CAD build for the part. Positions are in the model's coordinates, mm. Round coordinates to 2 decimals unless told otherwise and drop trailing zeros. Write each loop counter-clockwise with the first axis right and the second up, starting at its lowest first coordinate (ties: lowest second). Pieces come first, ordered by that corner, then holes. Notation, with made-up numbers: (76.25, 55) - (108.25, 55) arc R7 ccw to (108.25, 67) - close; hole circle Ø1 at (71, 10). An arc over 180 degrees is marked (long way). Answer in a Markdown table with one row per item.
Autodesk Inventor part; units mm, degrees
ref_plane "YZ Plane" through (0, 0, 0) normal (1, 0, 0) x (0, 1, 0)
ref_plane "XZ Plane" through (0, 0, 0) normal (0, 1, 0) x (-1, 0, 0)
ref_plane "XY Plane" through (0, 0, 0) normal (0, 0, 1) x (1, 0, 0)
sketch "Sketch1" plane through (0, 0, 0) normal (0, 1, 0) x (-1, 0, 0)
  circle A0 centre (64.977, -75.4393) radius 17
  line L0 (64.977, -75.4393) -> (99.977, -75.4393)
  line L1 (64.977, -75.4393) -> (47.477, -45.1285)
  line L2 (64.977, -75.4393) -> (47.477, -105.7502)
  circle A1 centre (47.477, -45.1285) radius 12
  circle A2 centre (99.977, -75.4393) radius 12
  circle A3 centre (47.477, -105.7502) radius 12
  circle A4 centre (47.477, -45.1285) radius 5.5
  circle A5 centre (99.977, -75.4393) radius 5.5
  circle A6 centre (47.477, -105.7502) radius 5.5
  line L3 (105.977, -65.047) -> (53.477, -34.7362)
  line L4 (35.477, -45.1285) -> (35.477, -105.7502)
  line L5 (53.477, -116.1425) -> (105.977, -85.8317)
  point P0 (0, 0)
  dimension "d0" = 120
  dimension "d1" = 120
  dimension "d2" = 120
  dimension "d3" = 35
  dimension "d5" = 34
  dimension "d6" = 35
  dimension "d7" = 35
  dimension "d8" = 24
  dimension "d9" = 24
  dimension "d10" = 24
  dimension "d11" = 11
  dimension "d13" = 11
  dimension "d14" = 11
extrude "Extrusion1" add sketch "Sketch1" along normal blind 10 contours L0 A2 L5 A3 L2 A0 | A0 L1 A1 L3 A2 L0 | A0 L2 A3 L4 A1 L1 | A2 | A1 | A3
equation "\"d1\" = d0"
equation "\"d6\" = d3"
equation "\"d7\" = d3"
equation "\"d9\" = d8"
equation "\"d10\" = d8"
equation "\"d13\" = d11"
Q1. Saw through at D-D on x = -64.5. List the corners of the cut face in (y, z).
Computed:
| item | result |
|---|---|
| outline | (0, -109.78) - (10, -109.78) - (10, -92.43) - (0, -92.43) - close; (0, -58.45) - (10, -58.45) - (10, -41.1) - (0, -41.1) - close |
Q2. Saw through at C-C on y = 2. List the corners of the cut face in (x, z).
Computed:
| item | result |
|---|---|
| outline | (-105.98, -85.83) - (-53.48, -116.14) arc R12 ccw to (-35.48, -105.75) - (-35.48, -45.13) arc R12 ccw to (-53.48, -34.74) - (-105.98, -65.05) arc R12 ccw to start; hole circle Ø11 at (-99.98, -75.44); hole circle Ø34 at (-64.98, -75.44); hole circle Ø11 at (-47.48, -105.75); hole circle Ø11 at (-47.48, -45.13) |
Q3. Saw through at A-A on x = -43. List the corners of the cut face in (y, z), then the cut area to 3 significant figures.
Computed:
| item | result |
|---|---|
| outline | (0, -116.88) - (10, -116.88) - (10, -108.94) - (0, -108.94) - close; (0, -102.56) - (10, -102.56) - (10, -48.32) - (0, -48.32) - close; (0, -41.93) - (10, -41.93) - (10, -33.99) - (0, -33.99) - close |
| area | 701 mm2 |
Q4. Saw through at B-B on z = -72.5. List the corners of the cut face in (x, y).
Computed:
| item | result |
|---|---|
| outline | (-111.61, 0) - (-104.63, 0) - (-104.63, 10) - (-111.61, 10) - close; (-95.33, 0) - (-81.72, 0) - (-81.72, 10) - (-95.33, 10) - close; (-48.23, 0) - (-35.48, 0) - (-35.48, 10) - (-48.23, 10) - close |
Q5. Drill centre lines: line 1 (X direction, y = 5.25, z = -49); line 2 (Z direction, x = -76, y = 1); line 3 (X direction, y = 2, z = -50). Where is each one in solid material? Low to high.
Computed:
| item | result |
|---|---|
| line 1 | x = -78.18 to -51.38, -43.57 to -35.48 |
| line 2 | z = -103.14 to -88.38, -62.5 to -47.74 |
| line 3 | x = -79.91 to -50.03, -44.92 to -35.48 |
Q6. Flat gauge pins, fed straight in: pin 1 (5 mm diameter, centred on x = -72, y = 8.5, fed in from -Z); pin 2 (1.5 mm diameter, centred on x = -99, y = 2, fed in from +Z); pin 3 (1.5 mm diameter, centred on y = 6.5, z = -70.5, fed in from -X). Where does each tip first touch, or does it go through?
Computed:
| item | result |
|---|---|
| pin 1 | stops at z = -106.89 |
| pin 2 | stops at z = -60.59 |
| pin 3 | stops at x = -111.22 |
Q7. Pull direction Z, two halves, no side cores. Call faces 1 (the flat face through (-47.7, 0, -74.8)), 2 (the cylindrical face through (-46.28, 4.93, -39.76)), 3 (the flat face through (-80.09, 4.93, -50.1)): released by +Z, released by -Z, zero draft, split by the parting line, or undercut.
Computed:
| item | result |
|---|---|
| face 1 | zero draft |
| face 2 | undercut |
| face 3 | released by +Z |
